Geometry: see drawing. Coordinates: mm, zero at the bounding-box minimum. Round coordinates to 2 decimals unless told otherwise and drop trailing zeros. Loops run counter-clockwise (first coordinate to the right, second up) from the corner with the lowest first, then second, coordinate; pieces in that order, holes last. Notation, with made-up numbers: (-40, 22) - (-31, 22) arc R23 ccw to (-31, 44) - close; hole circle Ø2 at (58, 26.25). An arc over 180 degrees is marked (long way). One line per question, with ' | ' between items. Start each with the question number.
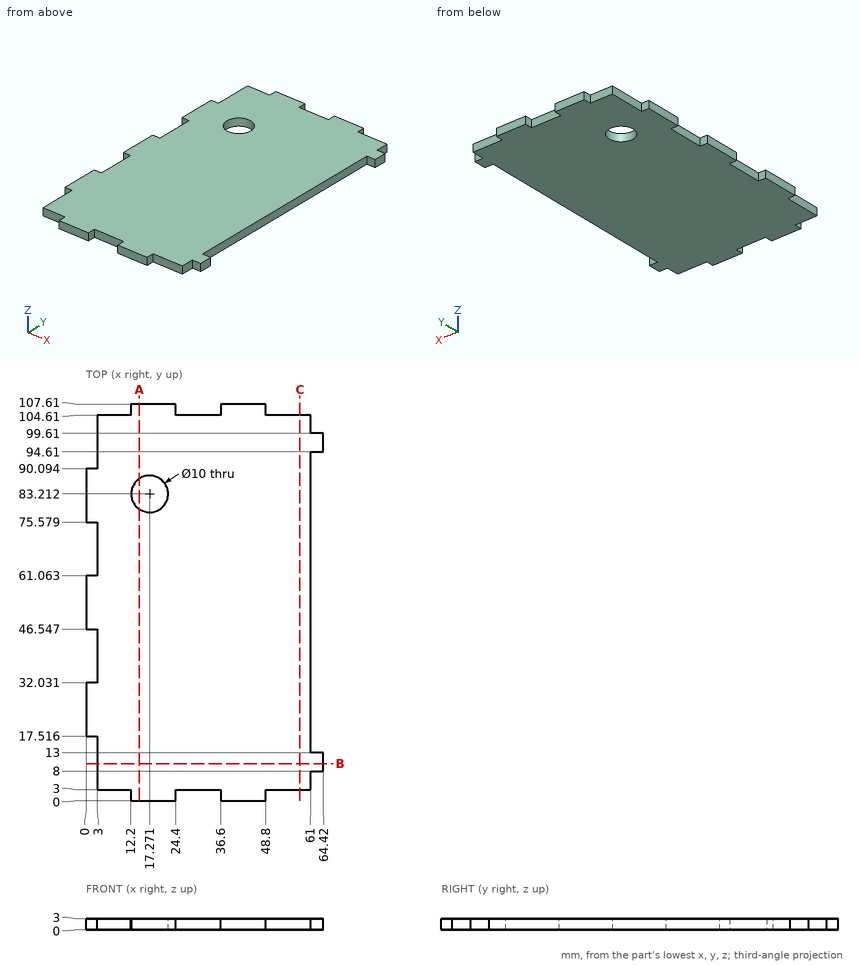
(1) Line query: line 1 along Y through (x, z) = (62, 0.3); line 2 along Y through (x, z) = (49, 0.95); line 3 along Y through (x, z) = (15.5, 2.6) (1 decimal). Output: solid intervals per line, ascending. Write a range as from..to.
(2) Section C-C, the plane x = 58. Output: boundary loops of the cut face in (y, z), plus the area to 3 significant figures.
(3) Section A-A, the plane x = 14.5. Output: boundary loops of the cut face in (y, z), plus the area to 3 significant figures.
(4) Section B-B, the plane y = 10. Output: boundary loops of the cut face in (x, z).
(5) Pin query (flat end, axial travel): P1, Ø1.5, axis at y = 102, z = 1.5, coming from the +X side; P2, Ø0.9, axis at x = 1.5, z = 2, coming from the -Y side; P3, Ø0.9, axis at y = 65.5, z = 1.5, coming from the -X side; P4, Ø1.5, axis at x = 54, y = 77, coming from the -Z side. Return the tip coordinate at first contact, or that it passes through.
Derived:
1) line 1: y = 8..13, 94.61..99.61 | line 2: y = 3..104.61 | line 3: y = 0..78.5, 87.9..107.6
2) outline: (3, 0) - (104.61, 0) - (104.61, 3) - (3, 3) - close | area: 305 mm²
3) outline: (0, 0) - (79.05, 0) - (79.05, 3) - (0, 3) - close; (87.37, 0) - (107.61, 0) - (107.61, 3) - (87.37, 3) - close | area: 298 mm²
4) outline: (3, 0) - (64.42, 0) - (64.42, 3) - (3, 3) - close
5) P1: stops at x = 61 | P2: stops at y = 17.52 | P3: stops at x = 3 | P4: stops at z = 0
